Design review of the part built by this model. Coordinates are the model's own, in mm. Face numbers are marked on the shaded views. A direction names the side the tool comes from. Give positions to 0.01 mm unless a question says otherwise; leave off trailing zeros. Order: outer loops, then holes, each group sorted by start corner. A loop starts at its lowest first (then second) coordinate and runs counter-clockwise, first axis right, second up. Notation, with made-up numbers: (-16, 15.25) -> (7, 15.25) arc R21 cw to (7, 19.25) -> close; hole circle Ø4 at (-0.75, 74.5). An arc over 180 degrees is marked (long way). One line per item, written item: value. Start each with the question number.
1) Consider section B-B (y = 0). State the section outline as (x, z) points, plus the area to 3 significant figures.
2) Tool access review of the marked faces 1 and 2: name each direction out of +Z, -Z, +X, -X, +Y, -Y from which nothing blocks a thin tool from reaching the whole face with its end or side.
3) Consider section D-D (z = -5.75). State the section outline as (x, y) points.
4) Wall thickness on line 1 along X through (y, z) = (1, -8); line 2 along X through (y, z) = (3.5, 1); line 3 along Y through (x, z) = (10.5, 0): over which ranges is each line inside the solid? List them lowest first. Write a range as from..to.
5) Consider section A-A (z = 0). State the section outline as (x, y) points.
6) For pin 1 (10 mm diameter, centred on x = 31.5, y = 3.5, fed in from -Z); pin 2 (1 mm diameter, centred on y = 6, z = 6.5, fed in from +X); pin 3 (5 mm diameter, centred on x = 15.5, z = 1.5, fed in from -Y), all flat-tipped, find the tip position at first contact; note any pin that passes through.
7) Consider section C-C (x = 26.5). State the section outline as (y, z) points.
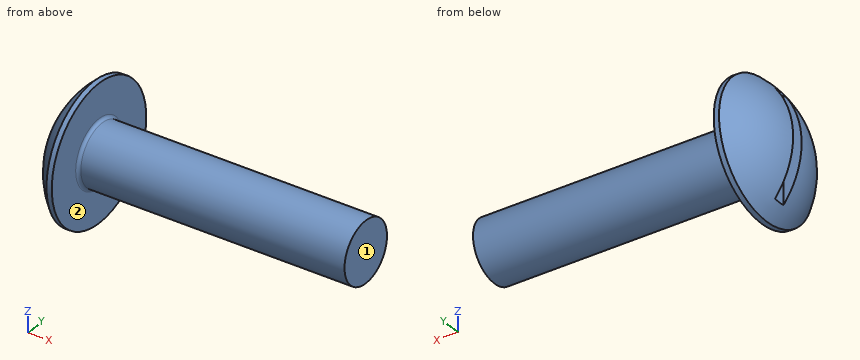
from build123d import *

# Parameters (mm, degrees)
FILLET1_R  = 0.4
SKETCH2_W  = 17.8
SKETCH2_H  = 1.6
SLOT_DEPTH = 2.4


with BuildPart() as part:
    # BodySke → Base-Revolve (revolve)
    with BuildSketch(Plane.XY, mode=Mode.PRIVATE) as base_revolve_sk:
        with BuildLine():
            Line((4.8, 4), (4.8, 8.9))
            Line((4.8, 8.9), (4.105264982, 8.9))
            ThreePointArc((4.105264982, 8.9), (1.075772976, 4.900591816), (0, 0))
            Line((0, 0), (39.8, 0))
            Line((39.8, 0), (39.8, 4))
            Line((39.8, 4), (4.8, 4))
        make_face()
    revolve(base_revolve_sk.sketch.rotate(Axis((-25.4, 0, 0), (1, 0, 0)), 90), axis=Axis((-25.4, 0, 0), (1, 0, 0)))

    # Fillet1
    fillet1_edges = [part.edges().sort_by_distance(p)[0] for p in [
        (4.8, 0, -4),
    ]]
    fillet(fillet1_edges, radius=FILLET1_R)

    # Sketch2 → Slot (cut)
    with BuildSketch(Plane(origin=(0, 0, 0), x_dir=(0, 0, -1), z_dir=(1, 0, 0))):
        Rectangle(SKETCH2_W, SKETCH2_H)
    extrude(amount=SLOT_DEPTH, mode=Mode.SUBTRACT)


solid = part.part
Checked values:
1. outline: (2.4, -7.1) arc R11.7 ccw to (4.11, -8.9) -> (4.8, -8.9) -> (4.8, -4.4) arc R0.4 cw to (5.2, -4) -> (39.8, -4) -> (39.8, 4) -> (5.2, 4) arc R0.4 cw to (4.8, 4.4) -> (4.8, 8.9) -> (4.11, 8.9) arc R11.7 ccw to (2.4, 7.1) -> close
1. area: 320 mm^2
2. face 1: +Z, -Z, +X, +Y, -Y
2. face 2: +X
3. outline: (1.54, -0.8) arc R10.19 ccw to (4.11, -6.79) -> (4.8, -6.79) -> (4.8, 6.79) -> (4.11, 6.79) arc R10.19 ccw to (1.54, 0.8) -> (2.4, 0.8) -> (2.4, -0.8) -> close
4. line 1: x = 3.22..4.8
4. line 2: x = 0.58..39.8
4. line 3: y = -4..4
5. outline: (0.03, -0.8) arc R11.7 ccw to (4.11, -8.9) -> (4.8, -8.9) -> (4.8, -4.4) arc R0.4 cw to (5.2, -4) -> (39.8, -4) -> (39.8, 4) -> (5.2, 4) arc R0.4 cw to (4.8, 4.4) -> (4.8, 8.9) -> (4.11, 8.9) arc R11.7 ccw to (0.03, 0.8) -> (2.4, 0.8) -> (2.4, -0.8) -> close
6. pin 1: stops at z = -4
6. pin 2: stops at x = 4.8
6. pin 3: stops at y = -4
7. outline: circle Ø8 at (0, 0)
